Autodesk Inventor part; units mm, degrees
ref_plane "YZ Plane" through (0, 0, 0) normal (1, 0, 0) x (0, 1, 0)
ref_plane "XZ Plane" through (0, 0, 0) normal (0, 1, 0) x (-1, 0, 0)
ref_plane "XY Plane" through (0, 0, 0) normal (0, 0, 1) x (1, 0, 0)
sketch "Sketch6" plane through (0, 0, 0) normal (0, 0, 1) x (1, 0, 0)
  line L0 (0, 0) -> (82.3, 0)
  line L1 (82.3, 0) -> (82.3, 20)
  line L2 (82.3, 20) -> (0, 20)
  line L3 (0, 20) -> (0, 0)
  line L4 (0, 0) -> (10, 0) construction
  line L5 (10, 0) -> (10, 26.8607) construction
  line L6 (0, 10) -> (82.8633, 10) construction
  line L7 (82.3, 0) -> (72.3, 0) construction
  line L8 (72.3, 0) -> (72.3, 17.2228) construction
  circle A0 centre (10, 10) radius 2.75
  circle A1 centre (72.3, 10) radius 2.75
  dimension "d32" = 82.3
  dimension "d33" = 20
  dimension "d34" = 10
  dimension "d35" = 10
  dimension "d36" = 5.5
  dimension "d37" = 5.5
extrude "Extrusion5" add sketch "Sketch6" along normal blind 5
sketch "Sketch7" plane through (0, 0, 0) normal (0, -1, 0) x (1, 0, 0)
  line L0 (82.3, 0) -> (82.3, 5)
  line L1 (0, 0) -> (0, 5)
  line L2 (41.15, 21.713) -> (41.15, -8.4757)
  line L3 (64.494, 5) -> (64.494, 55)
  line L4 (64.494, 55) -> (14.494, 55)
  line L5 (14.494, 55) -> (14.494, 5)
  line L6 (14.494, 5) -> (0, 5)
  line L7 (64.494, 5) -> (82.3, 5)
  line L8 (82.3, 0) -> (0, 0)
  dimension "d40" = 50
  dimension "d41" = 50
extrude "Extrusion6" add sketch "Sketch7" along normal blind 3
sketch "Sketch8" plane through (64.494, 0, 55) normal (1, 0, 0) x (0, 0, -1)
  line L0 (0, 0) -> (50, 0)
  line L1 (0, 0) -> (50, 19.8426)
  line L2 (0, 0) -> (50, 0)
  line L3 (50, 0) -> (50, 19.8426)
  point P0 (55, 0)
extrude "Extrusion7" add sketch "Sketch8" against normal blind 3
sketch "Sketch9" plane through (14.494, 0, 5) normal (-1, 0, 0) x (0, 0, 1)
  line L0 (50, 0) -> (50, -3)
  line L1 (0, 0) -> (50, 0)
  line L2 (50, 0) -> (0, 20.0433)
  line L3 (0, 0) -> (0, 20.0433)
extrude "Extrusion8" add sketch "Sketch9" against normal blind 3
sketch "Sketch10" plane through (0, 0, 0) normal (0, 1, 0) x (1, 0, 0)
  line L0 (17.494, -5) -> (61.494, -55) construction
  line L1 (61.494, -5) -> (17.494, -55) construction
  circle A0 centre (39.494, -30) radius 11.25
  circle A1 centre (39.494, -30) radius 12.25
  point P0 (0, 0)
  dimension "d48" = 22.5
  dimension "d49" = 24.5
extrude "Extrusion9" add sketch "Sketch10" along normal blind 7
sketch "Sketch11" plane through (39.494, 0, 30) normal (0, 1, 0) x (1, 0, 0)
  circle A0 centre (0, 0) radius 11.25
  circle A1 centre (0, 0) radius 5.4
  point P0 (-39.494, 30)
  dimension "d52" = 10.8
extrude "Extrusion10" cut sketch "Sketch11" against normal through all contours A1
properties part number "z leadscrew top mount" material "ABS Plastic"
Geometry check sheet. Reference: the model listing, model coordinates, mm. A direction names the side the tool comes from. Coordinates: 2 decimals unless noted, no trailing zeros. Order: outer loops, then holes, each group sorted by start corner. A loop starts at its lowest first (then second) coordinate and runs counter-clockwise, first axis right, second up. Notation, with made-up numbers: M 20,77 L 34,77 A7 ccw 34,84 Z; hole C 68.5,72 d1. An arc over 180 degrees is marked long. Use CSV: the item, a comma, the result in double quotes.
Item 1: Tool access check on faces 4 (the flat face through (17.494, 6, 19)), 5 (the flat face through (64.494, 6, 25)), 6 (the cylindrical face through (12.62, 9.17, 2.46)), 7 (the flat face through (34.3, 0, 41.5)). Record the directions out of +Z, -Z, +X, -X, +Y, -Y that give a thin tool (end or side, any length) a straight path to the whole face; none if there is none.
Returned:
face 4,"+Z, +Y"
face 5,"+Z, +X, +Y, -Y"
face 6,"+Z, -Z"
face 7,"+Y"
Item 2: Thickness scan on line 1 along X through (y, z) = (1.5, 30); line 2 along X through (y, z) = (12.5, 11); line 3 along X through (y, z) = (-0.75, 34). Record the ranges inside material, lowest first.
Returned:
line 1,"x = 14.49 to 17.49, 27.24 to 28.24, 50.74 to 51.74, 61.49 to 64.49"
line 2,"x = 14.49 to 17.49, 61.49 to 64.49"
line 3,"x = 14.49 to 35.87, 43.12 to 64.49"
Item 3: Cross-section at C-C on z = 30. Record the cut outline in (x, y), then the cut area to 3 significant figures.
Returned:
outline,"M 14.49,-3 L 34.09,-3 L 34.09,0 L 28.24,0 L 28.24,7 L 27.24,7 L 27.24,0 L 17.49,0 L 17.49,10.02 L 14.49,10.02 Z; M 44.89,-3 L 64.49,-3 L 64.49,9.92 L 61.49,9.92 L 61.49,0 L 51.74,0 L 51.74,7 L 50.74,7 L 50.74,0 L 44.89,0 Z"
area,"191 mm2"
Item 4: Cross-section at D-D on x = 16. Record the cut outline in (y, z), then the cut area to 3 significant figures.
Returned:
outline,"M -3,0 L 20,0 L 20,5 L 20.04,5 L 0,55 L -3,55 Z"
area,"766 mm2"
Item 5: Cross-section at A-A on x = 72.3. Record the cut outline in (y, z).
Returned:
outline,"M -3,0 L 7.25,0 L 7.25,5 L -3,5 Z; M 12.75,0 L 20,0 L 20,5 L 12.75,5 Z"
Item 6: Mould release check, pull along X, two halves, no side actions. Record for faces 1 (the flat face through (63.015, 9.782, 30.35)), 2 (the cylindrical face through (74.92, 9.17, 2.46)), 3 (the flat face through (14.494, 6, 24)): pulls with the +X half, pulls with the -X half, needs draft (parallel to the pull), parting line crosses it, or undercut.
Returned:
face 1,"needs draft"
face 2,"undercut"
face 3,"pulls with the -X half"
Item 7: Gauge pin test, flat ends, axial feed: pin 1 Ø22 at (x, z) = (39, 25.5) entering from +Y; pin 2 Ø2 at (x, y) = (37.5, 11) entering from +Z; pin 3 Ø6 at (y, z) = (6, 24.5) entering from -X. Record the tip position at first contact, or that the pin passes through.
Returned:
pin 1,"stops at y = 7"
pin 2,"stops at z = 5"
pin 3,"stops at x = 14.49"
Item 8: Cross-section at B-B on y = 1.5. Record the cut outline in (x, z), then the cut area to 3 significant figures.
Returned:
outline,"M 0,0 L 82.3,0 L 82.3,5 L 64.49,5 L 64.49,51.22 L 61.49,51.22 L 61.49,5 L 17.49,5 L 17.49,51.26 L 14.49,51.26 L 14.49,5 L 0,5 Z; C 39.49,30 d24.5; hole C 39.49,30 d22.5"
area,"763 mm2"
